Autodesk Inventor part; units mm, degrees
ref_plane "YZ Plane" through (0, 0, 0) normal (1, 0, 0) x (0, 1, 0)
ref_plane "XZ Plane" through (0, 0, 0) normal (0, 1, 0) x (-1, 0, 0)
ref_plane "XY Plane" through (0, 0, 0) normal (0, 0, 1) x (1, 0, 0)
sketch "Sketch1" plane through (0, 0, 0) normal (1, 0, 0) x (0, 1, 0)
  circle A0 centre (0, 0) radius 13.5
  dimension "d0" = 27
extrude "Extrusion1" add sketch "Sketch1" along normal blind 7
sketch "Sketch2" plane through (7, 0, 0) normal (1, 0, 0) x (0, 0, -1)
  circle A0 centre (0, 0) radius 7.5
  dimension "d3" = 15
extrude "Extrusion2" cut sketch "Sketch2" against normal blind 7
thread "Thread1"
sketch "Sketch3" plane through (7, 0, 0) normal (1, 0, 0) x (0, 0, -1)
  circle A0 centre (0, 0) radius 13.5
  line L0 (0, 13.5) -> (0, 11.5)
  line L1 (0, 11.5) -> (-2, 11.5)
  line L2 (-2, 11.5) -> (2, 11.5)
  line L3 (2, 11.5) -> (2, 14.5713)
  line L4 (2, 14.5713) -> (-2, 14.5713)
  line L5 (-2, 14.5713) -> (-2, 11.5)
  line L6 (-13.5, 0) -> (-11.5, 0)
  line L7 (-11.5, 0) -> (-11.5, -2)
  line L8 (-11.5, -2) -> (-11.5, 2)
  line L9 (-11.5, 2) -> (-14.5713, 2)
  line L10 (-14.5713, 2) -> (-14.5713, -2)
  line L11 (-14.5713, -2) -> (-11.5, -2)
  line L12 (0, -13.5) -> (0, -11.5)
  line L13 (0, -11.5) -> (2, -11.5)
  line L14 (2, -11.5) -> (-2, -11.5)
  line L15 (-2, -11.5) -> (-2, -14.5713)
  line L16 (-2, -14.5713) -> (2, -14.5713)
  line L17 (2, -14.5713) -> (2, -11.5)
  line L18 (13.5, 0) -> (11.5, 0)
  line L19 (11.5, 0) -> (11.5, 2)
  line L20 (11.5, 2) -> (11.5, -2)
  line L21 (11.5, -2) -> (14.5713, -2)
  line L22 (14.5713, -2) -> (14.5713, 2)
  line L23 (14.5713, 2) -> (11.5, 2)
  dimension "d8" = 2
  dimension "d9" = 2
  dimension "d10" = 4
  dimension "d13" = 360
extrude "Extrusion3" cut sketch "Sketch3" against normal blind 7 contours L18 L19 L23 A0 | A0 L23 L22 L21 | A0 L21 L20 L18 | L3 L2 L0 A0 | A0 L5 L4 L3 | L17 L16 L15 A0 | A0 L12 L13 L17 | L0 L1 L5 A0 | A0 L15 L14 L12 | L9 L8 L6 A0 | A0 L11 L10 L9 | A0 L6 L7 L11
properties part number "8. LockNutM15" material "Polyethylene, High Density"
Part model, mm, in its own coordinate system. A direction names the side the tool comes from. Coordinates: 2 decimals unless noted, no trailing zeros. Loops run counter-clockwise (first coordinate to the right, second up) from the corner with the lowest first, then second, coordinate; pieces in that order, holes last. Notation, with made-up numbers: (54, 32.25) - (62, 32.25) arc R9 ccw to (62, 36.25) - close; hole circle Ø1 at (62, 87.25). An arc over 180 degrees is marked (long way). Write item = value, one per line. Start each with the question number.
Item 1: Wall check: L1, parallel to Y at x = 4.25, z = 0; L2, parallel to Y at x = 2.25, z = 3; L3, parallel to Z at x = 1.5, y = 4.5. Give the ranges that are in metal, low to high. Write a range as from..to.
Item 2: 3-axis set-ups, long thin cutter, end or side, ignore diameter. For faces 1 (the flat face through (4, 0, 11.5)), 2 (the flat face through (4, 2, -12)), 3 (the flat face through (4, 12, -2)), 4 (the flat face through (4, -11.5, 0)): which of +Z, -Z, +X, -X, +Y, -Y reach the whole face in a straight line?
Item 3: Cut at D-D, the plane z = -9.25. Give the cut face in (x, y).
Item 4: Flat gauge pins, fed straight in: pin 1 Ø0.6 at (x, z) = (2, -12.5) entering from +Y; pin 2 Ø1.2 at (x, z) = (2, -0.5) entering from +Y; pin 3 Ø2 at (x, z) = (4, 12.5) entering from +Y; pin 4 Ø8 at (y, z) = (-4, -2.5) entering from +X. Where does each tip first touch, or does it go through?
Item 5: Cut at C-C, the plane x = 2. Give the cut face in (y, z), and give its area (3 significant figures).
Item 6: Cut at A-A, the plane y = 0. Give the cut face in (x, z).
Item 7: Mould opens along Z. For faces 5 (the flat face through (4, -12, -2)), 6 (the cylindrical face through (3.45, -9.63, 9.46)), 7 (the cylindrical face through (3.45, 9.63, -9.46)), 8 (the flat face through (4, 2, 12)) say: released by +Z, released by -Z, zero draft, split by the parting line, or undercut.
The answers:
q1.L1 = -11.5..-7.5, 7.5..11.5
q1.L2 = -13.16..-6.87, 6.87..13.16
q1.L3 = -12.73..-6, 6..12.73
q2.face_1 = +Z, +X, -X
q2.face_2 = -Z, +X, -X
q2.face_3 = +X, -X, +Y
q2.face_4 = +X, -X, -Y
q3.outline = (0, -9.83) - (7, -9.83) - (7, 9.83) - (0, 9.83) - close
q4.pin_1 = 5.78
q4.pin_2 = 11.5
q4.pin_3 = 7.07
q4.pin_4 = 7
q5.outline = (-13.35, -2) arc R13.5 ccw to (-2, -13.35) - (-2, -11.5) - (2, -11.5) - (2, -13.35) arc R13.5 ccw to (13.35, -2) - (11.5, -2) - (11.5, 2) - (13.35, 2) arc R13.5 ccw to (2, 13.35) - (2, 11.5) - (-2, 11.5) - (-2, 13.35) arc R13.5 ccw to (-13.35, 2) - (-11.5, 2) - (-11.5, -2) - close; hole circle Ø15 at (0, 0)
q5.area = 365 mm2
q6.outline = (0, -11.5) - (7, -11.5) - (7, -7.5) - (0, -7.5) - close; (0, 7.5) - (7, 7.5) - (7, 11.5) - (0, 11.5) - close
q7.face_5 = undercut
q7.face_6 = released by +Z
q7.face_7 = released by -Z
q7.face_8 = zero draft
